Design review of the part built by this model. Coordinates are the model's own, in mm. A direction names the side the tool comes from. Coordinates: 2 decimals unless noted, no trailing zeros. Write each loop counter-clockwise with the first axis right and the second up, starting at its lowest first coordinate (ties: lowest second). Pieces come first, ordered by that corner, then holes. Notation, with made-up numbers: M -36.75,63 L -32.75,63 A8 ccw -32.75,70 Z; hole C 58.25,88.5 d2. An arc over 180 degrees is marked long. Write item = value, one per line.
Autodesk Inventor part; units mm, degrees
ref_plane "YZ Plane" through (0, 0, 0) normal (1, 0, 0) x (0, 1, 0)
ref_plane "XZ Plane" through (0, 0, 0) normal (0, 1, 0) x (-1, 0, 0)
ref_plane "XY Plane" through (0, 0, 0) normal (0, 0, 1) x (1, 0, 0)
sketch "Sketch1" plane through (0, 0, 0) normal (0, 0, 1) x (1, 0, 0)
  line L0 (0, 0) -> (0, 54.375) construction
  line L1 (0, 54.375) -> (192, 54.375)
  line L2 (0, 0) -> (524.135, 0)
  line L3 (254.7886, 18.124) -> (254.7886, 0) construction
  line L4 (192, 54.375) -> (254.7886, 18.124)
  line L5 (254.7886, 18.124) -> (325.1228, 36.97)
  line L6 (325.1228, 36.97) -> (325.1228, 0) construction
  line L7 (192, 54.375) -> (192, 0) construction
  line L8 (325.1228, 51.4639) -> (256.7665, 33.1479)
  line L9 (256.7665, 33.1479) -> (195.7513, 68.375)
  line L10 (195.7513, 68.375) -> (0, 68.375)
  line L11 (0, 54.375) -> (0, 68.375)
  line L12 (325.1228, 36.97) -> (325.1228, 51.4639)
  line L13 (0, 68.375) -> (0, 73.375)
  line L14 (0, 73.375) -> (15, 73.375)
  line L15 (15, 73.375) -> (15, 68.375)
  line L16 (195.7513, 68.375) -> (195.7513, 73.375)
  line L17 (195.7513, 73.375) -> (180.7513, 73.375)
  line L18 (180.7513, 73.375) -> (180.7513, 68.375)
  dimension "d0" = 54.375
  dimension "d1" = 192
  dimension "d2" = 18.124
  dimension "d3" = 30
  dimension "d4" = 15
  dimension "d5" = 36.97
  dimension "d6" = 14
  dimension "d8" = 5
  dimension "d9" = 15
  dimension "d10" = 5
  dimension "d11" = 15
revolve "Revolution1" add sketch "Sketch1" angle 360 about axis through (0, 0, 0) along (1, 0, 0)
sketch "Sketch2" plane through (0, 0, 0) normal (-1, 0, 0) x (0, 0, 1)
  point P0 (0, 0)
properties part number "concept 2"
Q1. For P1, Ø8, axis at x = 73.5, y = -33.5, coming from the -Z side; P2, Ø6, axis at x = 60, z = 53, coming from the -Y side; P3, Ø5, axis at x = 105, z = -22, coming from the +Y side, all flat-tipped, find the tip position at first contact; note any pin that passes through.
Check result:
P1 = -61.68
P2 = -46.64
P3 = 65.54
Q2. Wall thickness on line 1 (Z direction, x = 98.5, y = 0) (3 decimals); line 2 (X direction, y = -46, z = 56); line 3 (Z direction, x = 216, y = -16): over which ranges is each line inside the solid? List them lowest first.
Check result:
line_1 = -68.375 to -54.375, 54.375 to 68.375
line_2 = 0 to 15, 180.75 to 195.75
line_3 = -54.38 to -37.23, 37.23 to 54.38
Q3. The part is to be moulded in two halves that separate along Y. For faces 1 (the flat face through (195.751, -60.1, 33)), 2 (the cylindrical face through (188.15, -15.91, 71.63)), 3 (the conical face through (236.908, -22.575, 17.31)), say which applies: +Y half, -Y half, draft (parallel to the pull), parting line (faces both ways), or undercut.
Check result:
face_1 = draft
face_2 = parting line
face_3 = undercut
Q4. Consider section C-C, the plane x = 91. State the section outline as (y, z) points (3 decimals).
Check result:
outline = C 0,0 d136.75; hole C 0,0 d108.75
Q5. Consider section A-A, the plane z = 0. State the section outline as (x, y) points (1 decimal).
Check result:
outline = M 0,-73.4 L 15,-73.4 L 15,-68.4 L 180.8,-68.4 L 180.8,-73.4 L 195.8,-73.4 L 195.8,-68.4 L 256.8,-33.1 L 325.1,-51.5 L 325.1,-37 L 254.8,-18.1 L 192,-54.4 L 0,-54.4 Z; M 0,54.4 L 192,54.4 L 254.8,18.1 L 325.1,37 L 325.1,51.5 L 256.8,33.1 L 195.8,68.4 L 195.8,73.4 L 180.8,73.4 L 180.8,68.4 L 15,68.4 L 15,73.4 L 0,73.4 Z
Q6. Consider section D-D, the plane x = 228. State the section outline as (y, z) points, and give its area (3 significant figures).
Check result:
outline = C 0,0 d99.51; hole C 0,0 d67.18
area = 4,230 mm²
Q7. Machinability: for faces 4 (the flat face through (15, -60.1, 33)), 5 (the flat face through (0, -55, 0)), 6 (the cylindrical face through (97.34, -11.79, -53.08)), which of the approach directions +Z, -Z, +X, -X, +Y, -Y give a long, thin tool a straight path to every point of the face, cutting with its end or side? Answer none if there is none.
Check result:
face_4 = none
face_5 = +Z, -Z, -X, +Y, -Y
face_6 = -X
